Input: part model. Units: mm. Frame: model coordinates. A direction names the side the tool comes from. Give positions to 0.01 mm unless a question says otherwise; leave off trailing zeros. Use CSV: the item, a comma, the result in double quotes. Start each with the question number.
Q1. Pin query (flat end, axial travel): pin 1 (3 mm diameter, centred on x = 15.08, z = 18.83, fed in from -Y). Return the tip coordinate at first contact, or that it passes through.
Q2. Pull-direction query (Z, two-part tool) for faces 1 (the flat face through (25, 1, 120.65)), 2 (the flat face through (15, 1, 45.53)), 3 (the flat face through (25, 0, 59)); classes: released by +Z, released by -Z, zero draft, split by the parting line, or undercut.
Q3. Material intervals for line 1 along X through (y, z) = (0.9, 51); line 2 along Z through (x, y) = (16, 0.75); line 3 along Z through (x, y) = (14.25, 2), sorted ascending.
Q4. Section A-A, the plane y = 1.3. State how many separate pieces and enclosed holes the cut face has, plus the area to 3 significant figures.
Q5. Reachability of faces 4 (the flat face through (11.43, 1, 61)), 5 (the flat face through (16.318, 1, 29)) from +Z, -Z, +X, -X, +Y, -Y: full face, straight path, thin tool, end or side. Return the list, or none.
from build123d import *

# Parameters (mm, degrees)
SKETCH1_W           = 19.05
SKETCH1_H           = 2.38125
BOSS_EXTRUDE1_DEPTH = 120.65
SKETCH8_W           = 19.05
SKETCH8_H           = 120.65
BOSS_EXTRUDE3_DEPTH = 2.38125
SKETCH9_R           = 1.905
CUT_EXTRUDE5_DEPTH  = 3.38125
SKETCH5_R           = 1.905
CUT_EXTRUDE6_DEPTH  = 2.54
SKETCH10_W          = 38.1
SKETCH10_H          = 29.6545
BOSS_EXTRUDE4_DEPTH = 2.38125
SKETCH12_W          = 11.43
SKETCH12_H          = 150.3045
CUT_EXTRUDE8_DEPTH  = 3.38125
SKETCH13_W          = 26.67
SKETCH13_H          = 29.6545
CUT_EXTRUDE9_DEPTH  = 3.38125


with BuildPart() as part:
    # Sketch1 → Boss-Extrude1 (new body)
    with BuildSketch(Plane.XY):
        with Locations((9.525, 1.190625)):
            Rectangle(SKETCH1_W, SKETCH1_H)
    extrude(amount=BOSS_EXTRUDE1_DEPTH)

    # Sketch8 → Boss-Extrude3 (add)
    with BuildSketch(Plane(origin=(0, 2.38125, 0), x_dir=(1, 0, 0), z_dir=(0, 1, 0))):
        with Locations((28.575, -60.325)):
            Rectangle(SKETCH8_W, SKETCH8_H)
    extrude(amount=-BOSS_EXTRUDE3_DEPTH)

    # Sketch9 → Cut-Extrude5 (cut, through all)
    with BuildSketch(Plane(origin=(0, 2.38125, 0), x_dir=(1, 0, 0), z_dir=(0, 1, 0))):
        with Locations((20.701, -114.5159)):
            Circle(SKETCH9_R)
    extrude(amount=-CUT_EXTRUDE5_DEPTH, mode=Mode.SUBTRACT)

    # Sketch5 → Cut-Extrude6 (cut)
    with BuildSketch(Plane(origin=(0, 2.38125, 0), x_dir=(1, 0, 0), z_dir=(0, 1, 0))):
        with Locations((15.08125, -39.14775)):
            Circle(SKETCH5_R)
        with Locations((15.08125, -18.82775)):
            Circle(SKETCH5_R)
        Polygon((16.317595, -28.98775), (16.317595, -32.5755), (15.08125, -32.5755), (13.844905, -32.5755), (13.844905, -25.2095), (16.317595, -25.2095), align=None)
        Polygon((15.08125, -52.8955), (16.317595, -52.8955), (16.317595, -45.5295), (13.844905, -45.5295), (13.844905, -52.8955), align=None)
    extrude(amount=-CUT_EXTRUDE6_DEPTH, mode=Mode.SUBTRACT)

    # Sketch10 → Boss-Extrude4 (add)
    with BuildSketch(Plane(origin=(0, 2.38125, 0), x_dir=(1, 0, 0), z_dir=(0, 1, 0))):
        with Locations((19.05, 14.82725)):
            Rectangle(SKETCH10_W, SKETCH10_H)
    extrude(amount=-BOSS_EXTRUDE4_DEPTH)

    # Sketch12 → Cut-Extrude8 (cut, through all)
    with BuildSketch(Plane(origin=(0, 2.38125, 0), x_dir=(1, 0, 0), z_dir=(0, 1, 0))):
        with Locations((5.715, -45.49775)):
            Rectangle(SKETCH12_W, SKETCH12_H)
    extrude(amount=-CUT_EXTRUDE8_DEPTH, mode=Mode.SUBTRACT)

    # Sketch13 → Cut-Extrude9 (cut, through all)
    with BuildSketch(Plane(origin=(0, 2.38125, 0), x_dir=(1, 0, 0), z_dir=(0, 1, 0))):
        with Locations((24.765, 14.82725)):
            Rectangle(SKETCH13_W, SKETCH13_H)
    extrude(amount=-CUT_EXTRUDE9_DEPTH, mode=Mode.SUBTRACT)


solid = part.part
A:
1,pin 1,"through"
2,face 1,"released by +Z"
2,face 2,"undercut"
2,face 3,"zero draft"
3,line 1,"11.43 to 13.84, 16.32 to 38.1"
3,line 2,"0 to 17.16, 20.5 to 25.21, 32.58 to 37.48, 40.82 to 45.53, 52.9 to 120.65"
3,line 3,"0 to 17.11, 20.54 to 25.21, 32.58 to 37.43, 40.86 to 45.53, 52.9 to 120.65"
4,separate pieces,"1"
4,enclosed holes,"5"
4,area,"3,150 mm^2"
5,face 4,"+Z, -Z, -X, +Y, -Y"
5,face 5,"+Y, -Y"
